Could you check a few things on this model? Use its own coordinates, in mm. Face numbers are marked on the shaded views. A direction names the side the tool comes from. Round coordinates to 2 decimals unless told otherwise and drop trailing zeros. Order: outer loops, then holes, each group sorted by start corner. A loop starts at its lowest first (then second) coordinate and runs counter-clockwise, first axis right, second up. Notation, with made-up numbers: (-3, -4.75) - (2, -4.75) arc R24 ccw to (2, 19.25) - close; hole circle Ø1 at (-0.75, 72). An arc over 180 degrees is marked (long way). Use one line per item in the form item = value.
from build123d import *

# Parameters (mm, degrees)
SALIENTE_EXTRUIR1_DEPTH = 12
SALIENTE_EXTRUIR2_DEPTH = 4.5
CORTAR_EXTRUIR1_DEPTH   = 17
REDONDEO1_R             = 1.5


with BuildPart() as part:
    # Croquis1 → Saliente-Extruir1 (new body)
    with BuildSketch(Plane.XY):
        with BuildLine():
            Line((-6.703786212, -4.139854541), (11.746213788, -4.139854541))
            Line((11.746213788, -4.139854541), (11.746213788, 4.160145459))
            Line((11.746213788, 4.160145459), (0.05, 4.160145459))
            Line((0.05, 4.160145459), (0.05, 5.660145459))
            Line((0.05, 5.660145459), (11.746213788, 5.660145459))
            ThreePointArc((11.746213788, 5.660145459), (12.806873959, 5.220805631), (13.246213788, 4.160145459))
            Line((13.246213788, 4.160145459), (13.246213788, -4.139854541))
            ThreePointArc((13.246213788, -4.139854541), (12.806873959, -5.200514713), (11.746213788, -5.639854541))
            Line((11.746213788, -5.639854541), (-11.803786212, -5.639854541))
            ThreePointArc((-11.803786212, -5.639854541), (-12.864446384, -5.200514713), (-13.303786212, -4.139854541))
            Line((-13.303786212, -4.139854541), (-13.303786212, 4.160145459))
            ThreePointArc((-13.303786212, 4.160145459), (-12.864446384, 5.220805631), (-11.803786212, 5.660145459))
            Line((-11.803786212, 5.660145459), (-0.05, 5.660145459))
            Line((-0.05, 5.660145459), (-0.05, 4.160145459))
            Line((-0.05, 4.160145459), (-11.803786212, 4.160145459))
            Line((-11.803786212, 4.160145459), (-11.803786212, -1.339854541))
            Line((-11.803786212, -1.339854541), (-6.703786212, -1.339854541))
            Line((-6.703786212, -1.339854541), (-6.703786212, -4.139854541))
        make_face()
    extrude(amount=SALIENTE_EXTRUIR1_DEPTH)

    # Croquis2 → Saliente-Extruir2 (add)
    with BuildSketch(Plane.XY.offset(12)):
        with BuildLine():
            Line((-11.803786212, -5.639854541), (11.746213788, -5.639854541))
            ThreePointArc((11.746213788, -5.639854541), (12.806873959, -5.200514713), (13.246213788, -4.139854541))
            Line((13.246213788, -4.139854541), (13.246213788, 4.160145459))
            ThreePointArc((13.246213788, 4.160145459), (12.806873959, 5.220805631), (11.746213788, 5.660145459))
            Line((11.746213788, 5.660145459), (0.05, 5.660145459))
            Line((0.05, 5.660145459), (0.05, 3.410145459))
            Line((0.05, 3.410145459), (10.996213788, 3.410145459))
            Line((10.996213788, 3.410145459), (10.996213788, -3.489854541))
            Line((10.996213788, -3.489854541), (-5.953786212, -3.489854541))
            Line((-5.953786212, -3.489854541), (-5.953786212, -0.589854541))
            Line((-5.953786212, -0.589854541), (-11.053786212, -0.589854541))
            Line((-11.053786212, -0.589854541), (-11.053786212, 3.410145459))
            Line((-11.053786212, 3.410145459), (-10.745057731, 3.410145459))
            Line((-10.745057731, 3.410145459), (-0.05, 3.410145459))
            Line((-0.05, 3.410145459), (-0.05, 5.660145459))
            Line((-0.05, 5.660145459), (-11.803786212, 5.660145459))
            ThreePointArc((-11.803786212, 5.660145459), (-12.864446384, 5.220805631), (-13.303786212, 4.160145459))
            Line((-13.303786212, 4.160145459), (-13.303786212, -4.139854541))
            ThreePointArc((-13.303786212, -4.139854541), (-12.864446384, -5.200514713), (-11.803786212, -5.639854541))
        make_face()
    extrude(amount=SALIENTE_EXTRUIR2_DEPTH)

    # Croquis3 → Cortar-Extruir1 (cut)
    with BuildSketch(Plane(origin=(0, 0, 0), x_dir=(-1, 0, 0), z_dir=(0, 0, -1))):
        with BuildLine():
            Line((7.425674431, -5.454722367), (12.525674431, -2.654722367))
            ThreePointArc((12.525674431, -2.654722367), (13.094683638, -2.103781132), (13.303786212, -1.339854541))
            Line((13.303786212, -1.339854541), (14.985773561, -1.339854541))
            Line((14.985773561, -1.339854541), (14.985773561, -7.3319768))
            Line((14.985773561, -7.3319768), (6.703786212, -7.3319768))
            Line((6.703786212, -7.3319768), (6.703786212, -5.639854541))
            ThreePointArc((6.703786212, -5.639854541), (7.076410863, -5.592834537), (7.425674431, -5.454722367))
        make_face()
    extrude(amount=-CORTAR_EXTRUIR1_DEPTH, mode=Mode.SUBTRACT)

    # Redondeo1
    redondeo1_edges = [part.edges().sort_by_distance(p)[0] for p in [
        (12.806873959, -5.200514713, 16.5),
        (13.246213788, 0.010145459, 16.5),
        (12.806873959, 5.220805631, 16.5),
        (5.898106894, 5.660145459, 16.5),
        (-5.926893106, 5.660145459, 16.5),
        (-12.864446384, 5.220805631, 16.5),
        (-13.303786212, 1.410145459, 16.5),
        (2.521213788, -5.639854541, 16.5),
        (-13.094683638, -2.103781132, 16.5),
        (-9.975674431, -4.054722367, 16.5),
        (-7.076410863, -5.592834537, 16.5),
    ]]
    fillet(redondeo1_edges, radius=REDONDEO1_R)


solid = part.part
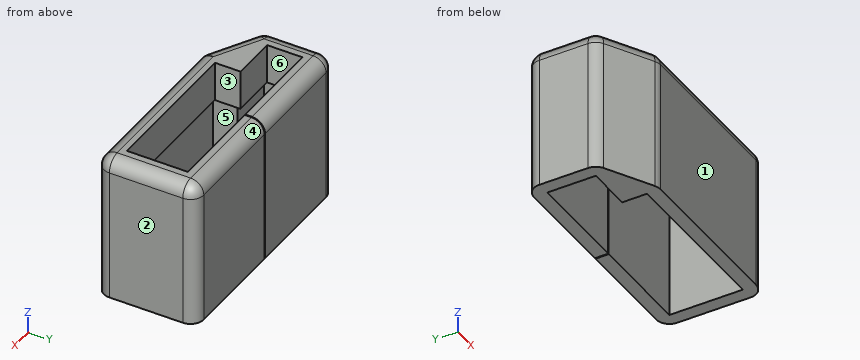
Item 1: I need wall thicknesses on L1, parallel to Y at x = 10, z = 6.25; L2, parallel to X at y = 1.25, z = 4; L3, parallel to Y at x = 4, z = 14.75. Which ranges of each line are inside material? Lowest first, please.
Found:
L1 = -5.64 to -4.14, 4.16 to 5.66
L2 = -13.3 to -11.8, 11.75 to 13.25
L3 = -5.64 to -3.49, 3.41 to 5.66
Item 2: Imagine slicing it at C-C on z = 11. Please give me the cut outline in (x, y).
Found:
outline = (-13.3, -1.34) arc R1.5 ccw to (-12.53, -2.65) - (-7.43, -5.45) arc R1.5 ccw to (-6.7, -5.64) - (11.75, -5.64) arc R1.5 ccw to (13.25, -4.14) - (13.25, 4.16) arc R1.5 ccw to (11.75, 5.66) - (0.05, 5.66) - (0.05, 4.16) - (11.75, 4.16) - (11.75, -4.14) - (-6.7, -4.14) - (-6.7, -1.34) - (-11.8, -1.34) - (-11.8, 4.16) - (-0.05, 4.16) - (-0.05, 5.66) - (-11.8, 5.66) arc R1.5 ccw to (-13.3, 4.16) - close
Item 3: Imagine slicing it at A-A on x = 4. Please give me the cut outline in (y, z).
Found:
outline = (-5.64, 0) - (-4.14, 0) - (-4.14, 12) - (-3.49, 12) - (-3.49, 16.5) - (-4.14, 16.5) arc R1.5 ccw to (-5.64, 15) - close; (3.41, 12) - (4.16, 12) - (4.16, 0) - (5.66, 0) - (5.66, 15) arc R1.5 ccw to (4.16, 16.5) - (3.41, 16.5) - close
Item 4: Will these pins go through, and if not, where does the flat tip stop? P1, Ø3, axis at x = -2.5, y = 0.5, coming from the +Z side; P2, Ø1, axis at y = -3, z = 5, coming from the -X side.
Found:
P1 = through
P2 = -12.75
Item 5: Imagine slicing it at B-B on y = 2. Please give me the cut outline in (x, z), plus the area to 3 significant figures.
Found:
outline = (-13.3, 0) - (-11.8, 0) - (-11.8, 12) - (-11.05, 12) - (-11.05, 16.5) - (-11.8, 16.5) arc R1.5 ccw to (-13.3, 15) - close; (11, 12) - (11.75, 12) - (11.75, 0) - (13.25, 0) - (13.25, 15) arc R1.5 ccw to (11.75, 16.5) - (11, 16.5) - close
area = 55.3 mm2
Item 6: If we mould it in two halves opening along X, with no side actions, what happens to the marked faces 1, 2 and 3? For each: released by +X, released by -X, zero draft, split by the parting line, or undercut.
Found:
face_1 = zero draft
face_2 = released by +X
face_3 = undercut
Item 7: For the marked faces 4, 5 and 6, which set-ups out of +Z, -Z, +X, -X, +Y, -Y let a thin tool reach every point of the face, with its end or its side?
Found:
face_4 = +Z, +X, -X, +Y
face_5 = -Z
face_6 = +Z, -Z
